from build123d import *

# Parameters (mm, degrees)
SKETCH_1_R          = 5.05
SKETCH_1_R_2        = 13
EXTRUDE_1_DEPTH     = 15
FILLET_1_R          = 3
CUT_EXTRUDE_3_DEPTH = 277.54113618
FILLET_2_R          = 3
EXTRUDE_START       = -15
SKETCH_5_R          = 27.5
SKETCH_5_R_2        = 5.05
EXTRUDE_2_DEPTH     = 15
FILLET_3_R          = 6
EXTRUDE_3_DEPTH     = 15
FILLET_4_R          = 3
SKETCH_7_R          = 2.05
CUT_EXTRUDE_4_DEPTH = 277.778340916
SKETCH_8_R          = 15
CUT_EXTRUDE_5_DEPTH = 277.778340916


with BuildPart() as part:
    # 草图1 → 凸台-拉伸1 (new body)
    with BuildSketch(Plane(origin=(0, 0, 0), x_dir=(1, 0, 0), z_dir=(0, 1, 0))):
        with BuildLine():
            Line((-17.992942616, -0.504), (-24.990198078, 249.3))
            ThreePointArc((-24.990198078, 249.3), (0, 275), (24.990198078, 249.3))
            Line((24.990198078, 249.3), (17.992942616, -0.504))
            ThreePointArc((17.992942616, -0.504), (0, -18), (-17.992942616, -0.504))
        make_face()
        with Locations(Location((0, 0, 0), (0, 0, 270))):
            Circle(SKETCH_1_R, mode=Mode.SUBTRACT)
        with Locations(Location((0, 250, 0), (0, 0, 270))):
            Circle(SKETCH_1_R_2, mode=Mode.SUBTRACT)
        Polygon((-16.444447487, 158.5), (-17.704941698, 203.5), (11.028871219, 137.174942267), align=None, mode=Mode.SUBTRACT)
        Polygon((15.954255294, 141), (18.475243716, 231), (-12, 219.5), align=None, mode=Mode.SUBTRACT)
    extrude(amount=EXTRUDE_1_DEPTH)

    # 圆角1
    fillet_1_edges = [part.edges().sort_by_distance(p)[0] for p in [
        (-16.444447487, 7.5, -158.5),
        (11.028871219, 7.5, -137.174942267),
        (-17.704941698, 7.5, -203.5),
        (18.475243716, 7.5, -231),
        (-12, 7.5, -219.5),
        (15.954255294, 7.5, -141),
    ]]
    fillet(fillet_1_edges, radius=FILLET_1_R)

    # 草图4 → 切除-拉伸3 (cut, through all)
    with BuildSketch(Plane(origin=(0, 15, 0), x_dir=(1, 0, 0), z_dir=(0, 1, 0))):
        Polygon((-13.050343026, 144.472367448), (12.494927596, 124.643879429), (9.742058902, 26.365688077), (-10.175105816, 41.825585442), align=None)
    extrude(amount=-CUT_EXTRUDE_3_DEPTH, mode=Mode.SUBTRACT)

    # 圆角2
    fillet_2_edges = [part.edges().sort_by_distance(p)[0] for p in [
        (-10.175105816, 7.5, -41.825585442),
        (-13.050343026, 7.5, -144.472367448),
        (9.742058902, 7.5, -26.365688077),
    ]]
    fillet(fillet_2_edges, radius=FILLET_2_R)

    # 草图5 → 凸台-拉伸2 (add)
    with BuildSketch(Plane(origin=(0, 15, 0), x_dir=(1, 0, 0), z_dir=(0, 1, 0)).offset(EXTRUDE_START)):
        Circle(SKETCH_5_R)
        with Locations(Location((0, 0, 0), (0, 0, 270))):
            Circle(SKETCH_5_R_2, mode=Mode.SUBTRACT)
    extrude(amount=EXTRUDE_2_DEPTH)

    # 圆角3
    fillet_3_edges = [part.edges().sort_by_distance(p)[0] for p in [
        (-18.575080057, 7.5, -20.278471364),
        (18.575080057, 7.5, -20.278471364),
    ]]
    fillet(fillet_3_edges, radius=FILLET_3_R)

    # 草图6 → 凸台-拉伸3 (add)
    with BuildSketch(Plane(origin=(0, 15, 0), x_dir=(1, 0, 0), z_dir=(0, 1, 0))):
        Polygon((9.60137553, 125.435937788), (-13.068657882, 42.617643801), (-7.609801347, 39.834371112), (-7.28155375, 41.033527083), (15.388479662, 123.85182107), (9.929623127, 126.635093759), align=None)
    extrude(amount=-EXTRUDE_3_DEPTH)

    # 圆角4
    fillet_4_edges = [part.edges().sort_by_distance(p)[0] for p in [
        (9.929623127, 7.5, -126.635093759),
        (12.14036175, 7.5, -111.985778385),
        (-7.609801347, 7.5, -39.834371112),
        (-10.463842583, 7.5, -52.133569747),
    ]]
    fillet(fillet_4_edges, radius=FILLET_4_R)

    # 草图7 → 切除-拉伸4 (cut, through all)
    with BuildSketch(Plane(origin=(0, 15, 0), x_dir=(1, 0, 0), z_dir=(0, 1, 0))):
        with Locations(Location((15, 15, 0), (0, 0, 270))):
            Circle(SKETCH_7_R)
        with Locations(Location((-15, 15, 0), (0, 0, 270))):
            Circle(SKETCH_7_R)
        with Locations(Location((-15, -15, 0), (0, 0, 270))):
            Circle(SKETCH_7_R)
        with Locations(Location((15, -15, 0), (0, 0, 270))):
            Circle(SKETCH_7_R)
    extrude(amount=-CUT_EXTRUDE_4_DEPTH, mode=Mode.SUBTRACT)

    # 草图8 → 切除-拉伸5 (cut, through all)
    with BuildSketch(Plane(origin=(0, 15, 0), x_dir=(1, 0, 0), z_dir=(0, 1, 0))):
        with Locations(Location((0, 0, 0), (0, 0, 270))):
            Circle(SKETCH_8_R)
    extrude(amount=-CUT_EXTRUDE_5_DEPTH, mode=Mode.SUBTRACT)


solid = part.part
Can you work these out from the model? Positions are in its coordinate system, mm. Coordinates: 2 decimals unless noted, no trailing zeros. Write each loop counter-clockwise with the first axis right and the second up, starting at its lowest first coordinate (ties: lowest second). Pieces come first, ordered by that corner, then holes. Notation, with made-up numbers: M -11,67 L 6,67 A16 ccw 6,81 Z; hole C -34.75,-22 d5. An arc over 180 degrees is marked long. Use one line per item in the form item = value.
Q1. If we section it at D-D (z = -255): Write out the boundary of the cut face in (x, y), then the cut area to 3 significant figures.
Model answer:
outline = M -24.49,0 L -12,0 L -12,15 L -24.49,15 Z; M 12,0 L 24.49,0 L 24.49,15 L 12,15 Z
area = 375 mm^2
Q2. If we section it at B-B (z = -82.5): Write out the boundary of the cut face in (x, y).
Model answer:
outline = M -20.32,0 L -11.31,0 L -11.31,15 L -20.32,15 Z; M -2.15,0 L 4.07,0 L 4.07,15 L -2.15,15 Z; M 11.31,0 L 20.32,0 L 20.32,15 L 11.31,15 Z
Q3. For P1, Ø4, axis at x = 6, y = 6.5, coming from the -Z side; P2, Ø2, axis at x = -16.5, y = 5.5, coming from the +Z side; P3, Ø5, axis at y = 13, z = -179.5, coming from the -X side, each with a flat end and sliding along its axis, tell me the tip position at first contact or that it passes through.
Model answer:
P1 = -274.68
P2 = 22.72
P3 = -23.11
Q4. We'd pull the mould along Z, two halves only. Please class faces 1 (the flat face through (-13, 15, -126)), 2 (the flat face through (0.04, 7.61, -134.31)): +Z half, -Z half, draft (parallel to the pull), parting line (faces both ways), or undercut.
Model answer:
face_1 = draft
face_2 = undercut
Q5. If we section it at C-C (y = 8.5): State how many separate pieces and enclosed holes the cut face has, then the cut area to 3 significant figures.
Model answer:
separate_pieces = 1
enclosed_holes = 10
area = 8,370 mm^2
Q6. If we section it at A-A (z = 0): Write out the boundary of the cut face in (x, y).
Model answer:
outline = M -27.5,0 L -15,0 L -15,15 L -27.5,15 Z; M 15,0 L 27.5,0 L 27.5,15 L 15,15 Z
Q7. I need wall thicknesses on line 1 along X through (y, z) = (9, 0); line 2 along X through (y, z) = (8.5, -82.5); line 3 along X through (y, z) = (5.75, -162). Which ranges of each line are inside material? Lowest first, please. Write a range as from..to.
Model answer:
line_1 = -27.5..-15, 15..27.5
line_2 = -20.32..-11.31, -2.15..4.07, 11.31..20.32
line_3 = -22.54..-16.54, 0.27..8.48, 16.54..22.54
